Model file for the job. Use its own axes, mm. A direction names the side the tool comes from. Coordinates: 2 decimals unless noted, no trailing zeros. Write each loop counter-clockwise with the first axis right and the second up, starting at its lowest first coordinate (ties: lowest second). Pieces come first, ordered by that corner, then holes. Notation, with made-up numbers: (60.5, -32.75) -> (111.5, -32.75) arc R24 cw to (111.5, -5.75) -> close; hole circle Ø9 at (-20.75, 39). An arc over 180 degrees is marked (long way). Answer as a JSON object with one key per item and string values. Group by question number.
from build123d import *

# Parameters (mm, degrees)
F0_R     = 5
F1_DEPTH = 10
F2_D     = 10
F3_D     = 10
F4_D     = 10
F5_D     = 10
F6_DEPTH = 20
F8_D     = 17.5


with BuildPart() as f1:
    # F0 (on Top) → F1 (new body)
    with BuildSketch(Plane.XY):
        with BuildLine():
            Line((0, 30), (-20, 30))
            ThreePointArc((-20, 30), (-27.0710678119, 27.0710678119), (-30, 20))
            Line((-30, 20), (-30, 0))
            Line((-30, 0), (-16, 0))
            ThreePointArc((-16, 0), (-11.313708499, 11.313708499), (0, 16))
            Line((0, 16), (0, 30))
        make_face()
        with Locations((-20, 20)):
            Circle(F0_R, mode=Mode.SUBTRACT)
        with BuildLine():
            Line((20, 30), (0, 30))
            Line((0, 30), (0, 16))
            ThreePointArc((0, 16), (11.313708499, 11.313708499), (16, 0))
            Line((16, 0), (30, 0))
            Line((30, 0), (30, 20))
            ThreePointArc((30, 20), (27.0710678119, 27.0710678119), (20, 30))
        make_face()
        with Locations((20, 20)):
            Circle(F0_R, mode=Mode.SUBTRACT)
        with BuildLine():
            Line((-16, 0), (-30, 0))
            Line((-30, 0), (-30, -20))
            ThreePointArc((-30, -20), (-27.0710678119, -27.0710678119), (-20, -30))
            Line((-20, -30), (0, -30))
            Line((0, -30), (0, -16))
            ThreePointArc((0, -16), (-11.313708499, -11.313708499), (-16, 0))
        make_face()
        with Locations((-20, -20)):
            Circle(F0_R, mode=Mode.SUBTRACT)
        with BuildLine():
            Line((30, 0), (16, 0))
            ThreePointArc((16, 0), (11.313708499, -11.313708499), (0, -16))
            Line((0, -16), (0, -30))
            Line((0, -30), (20, -30))
            ThreePointArc((20, -30), (27.0710678119, -27.0710678119), (30, -20))
            Line((30, -20), (30, 0))
        make_face()
        with Locations((20, -20)):
            Circle(F0_R, mode=Mode.SUBTRACT)
        with BuildLine():
            Line((0, 0), (0, 16))
            ThreePointArc((0, 16), (-11.313708499, 11.313708499), (-16, 0))
            Line((-16, 0), (0, 0))
        make_face()
        with BuildLine():
            ThreePointArc((16, 0), (11.313708499, 11.313708499), (0, 16))
            Line((0, 16), (0, 0))
            Line((0, 0), (16, 0))
        make_face()
        with BuildLine():
            ThreePointArc((0, -16), (11.313708499, -11.313708499), (16, 0))
            Line((16, 0), (0, 0))
            Line((0, 0), (0, -16))
        make_face()
        with Locations((-20, 20)):
            Circle(F0_R)
        with Locations((20, 20)):
            Circle(F0_R)
        with BuildLine():
            Line((0, 0), (-16, 0))
            ThreePointArc((-16, 0), (-11.313708499, -11.313708499), (0, -16))
            Line((0, -16), (0, 0))
        make_face()
        with Locations((20, -20)):
            Circle(F0_R)
        with Locations((-20, -20)):
            Circle(F0_R)
    extrude(amount=-F1_DEPTH)

    # F2 (through all)
    with Locations(Plane.XY):
        with Locations((-20, 20)):
            Hole(F2_D / 2)

    # F3 (through all)
    with Locations(Plane.XY):
        with Locations((20, 20)):
            Hole(F3_D / 2)

    # F4 (through all)
    with Locations(Plane.XY):
        with Locations((20, -20)):
            Hole(F4_D / 2)

    # F5 (through all)
    with Locations(Plane.XY):
        with Locations((-20, -20)):
            Hole(F5_D / 2)

    # F0 (on Top) → F6 (join)
    with BuildSketch(Plane.XY):
        with BuildLine():
            Line((0, 0), (0, 16))
            ThreePointArc((0, 16), (-11.313708499, 11.313708499), (-16, 0))
            Line((-16, 0), (0, 0))
        make_face()
        with BuildLine():
            ThreePointArc((16, 0), (11.313708499, 11.313708499), (0, 16))
            Line((0, 16), (0, 0))
            Line((0, 0), (16, 0))
        make_face()
        with BuildLine():
            ThreePointArc((0, -16), (11.313708499, -11.313708499), (16, 0))
            Line((16, 0), (0, 0))
            Line((0, 0), (0, -16))
        make_face()
        with BuildLine():
            Line((0, 0), (-16, 0))
            ThreePointArc((-16, 0), (-11.313708499, -11.313708499), (0, -16))
            Line((0, -16), (0, 0))
        make_face()
    extrude(amount=F6_DEPTH)

    # F8 (through all)
    with Locations(Plane.XY.offset(20)):
        with Locations((0, 0)):
            Hole(F8_D / 2)


solid = f1.part
(1) Cut at B-B on y = 21. List the corners of the cut face in (x, z), plus the area to 3 significant figures.
(2) Wall check: probe 1 along Y at (x, z) = (20, -6.25); probe 2 along Y at (x, z) = (-18, -2); probe 3 along Z at (x, y) = (-23.5, -8.5). Give the ranges that are in metal, low to high.
(3) Cut at A-A on y = -2.5. List the corners of the cut face in (x, z), plus the area to 3 significant figures.
(4) Pin check, flat tips, straight feed: pin 1 (4 mm diameter, centred on y = -6.5, z = 5, fed in from -X); pin 2 (2 mm diameter, centred on x = -22.5, y = -7, fed in from +Z). Stop position of each tip, or through.
(5) Cut at D-D on y = 13.5. List the corners of the cut face in (x, z).
(6) Cut at C-C on x = 7. List the corners of the cut face in (y, z), plus the area to 4 significant figures.
(7) Pull direction X, two halves, no side cores. Call faces 3 (the face through (30, 0, -5)), 4 (the face through (-27.15, -26.99, -4.93)), 5 (the face through (21.08, -24.88, -5.07)): released by +X, released by -X, zero draft, split by the parting line, or undercut.
(8) 3-axis set-ups, long thin cutter, end or side, ignore diameter. For faces 1 (the face through (-30, 0, -5)), 2 (the face through (13, -13, 0)): which of +Z, -Z, +X, -X, +Y, -Y reach the whole face in a straight line?
Results found:
{
 "1": {"outline": "(-29.95, -10) -> (-24.9, -10) -> (-24.9, 0) -> (-29.95, 0) -> close; (-15.1, -10) -> (15.1, -10) -> (15.1, 0) -> (-15.1, 0) -> close; (24.9, -10) -> (29.95, -10) -> (29.95, 0) -> (24.9, 0) -> close", "area": "403 mm²"},
 "2": {"probe 1": "y = -30 to -25, -15 to 15, 25 to 30", "probe 2": "y = -30 to -24.58, -15.42 to 15.42, 24.58 to 30", "probe 3": "z = -10 to 0"},
 "3": {"outline": "(-30, -10) -> (-8.39, -10) -> (-8.39, 20) -> (-15.8, 20) -> (-15.8, 0) -> (-30, 0) -> close; (8.39, -10) -> (30, -10) -> (30, 0) -> (15.8, 0) -> (15.8, 20) -> (8.39, 20) -> close", "area": "729 mm²"},
 "4": {"pin 1": "stops at x = -15.35", "pin 2": "stops at z = 0"},
 "5": {"outline": "(-30, -10) -> (30, -10) -> (30, 0) -> (8.59, 0) -> (8.59, 20) -> (-8.59, 20) -> (-8.59, 0) -> (-30, 0) -> close"},
 "6": {"outline": "(-30, -10) -> (-5.25, -10) -> (-5.25, 20) -> (-14.39, 20) -> (-14.39, 0) -> (-30, 0) -> close; (5.25, -10) -> (30, -10) -> (30, 0) -> (14.39, 0) -> (14.39, 20) -> (5.25, 20) -> close", "area": "860.5 mm²"},
 "7": {"face 3": "released by +X", "face 4": "released by -X", "face 5": "undercut"},
 "8": {"face 1": "+Z, -Z, -X, +Y, -Y", "face 2": "+Z"}
}
